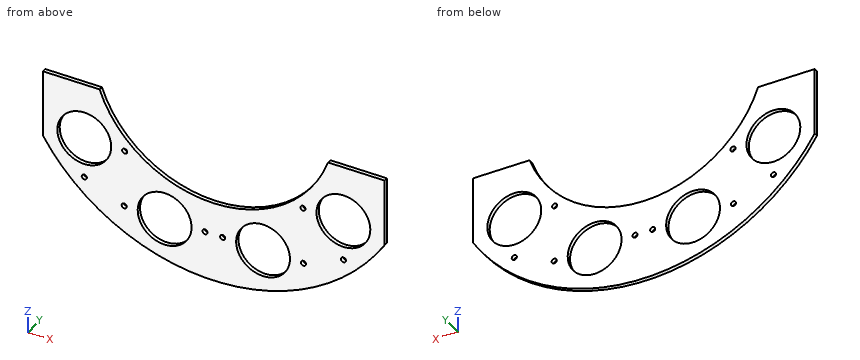
```python
from build123d import *

# Parameters (mm, degrees)
SKETCH3_R              = 20
BOSS_EXTRUDE3_DEPTH    = 3
F_10_24_TAPPED_HOLE1_D = 3.7973


with BuildPart() as part:
    # Sketch3 → Boss-Extrude3 (new body)
    with BuildSketch(Plane(origin=(0, 0, 0), x_dir=(1, 0, 0), z_dir=(0, 1, 0))):
        with BuildLine():
            Line((-126.885775404, -16.789832489), (-84.87168845, -16.789832489))
            ThreePointArc((-84.87168845, -16.789832489), (0, 43.227962976), (84.87168845, -16.789832489))
            Line((84.87168845, -16.789832489), (126.885775404, -16.789832489))
            Line((126.885775404, -16.789832489), (126.885775404, 33.210167511))
            ThreePointArc((126.885775404, 33.210167511), (0, 103.210167511), (-126.885775404, 33.210167511))
            Line((-126.885775404, 33.210167511), (-126.885775404, -16.789832489))
        make_face()
        with Locations(Location((-36.555626875, 67.506651026, 0), (0, 0, 270))):
            Circle(SKETCH3_R, mode=Mode.SUBTRACT)
        with Locations(Location((-96.223855306, 24.910723088, 0), (0, 0, 270))):
            Circle(SKETCH3_R, mode=Mode.SUBTRACT)
        with Locations(Location((36.555626875, 67.506651026, 0), (0, 0, 270))):
            Circle(SKETCH3_R, mode=Mode.SUBTRACT)
        with Locations(Location((96.223855306, 24.910723088, 0), (0, 0, 270))):
            Circle(SKETCH3_R, mode=Mode.SUBTRACT)
    extrude(amount=BOSS_EXTRUDE3_DEPTH)

    # #10-24 Tapped Hole1 (through all)
    with Locations(Plane(origin=(0, 3, 0), x_dir=(1, 0, 0), z_dir=(0, 1, 0))):
        with Locations((-66.223855306, 24.910723088), (-96.223855306, 54.910723088), (-66.555626875, 67.506651026), (-6.555626875, 67.506651026), (6.555626875, 67.506651026), (66.555626875, 67.506651026), (96.223855306, 54.910723088), (66.223855306, 24.910723088)):
            Hole(F_10_24_TAPPED_HOLE1_D / 2)


solid = part.part
```
CAD build for the part. Positions are in the model's coordinates, mm. Coordinates: 2 decimals unless noted, no trailing zeros. Loops run counter-clockwise (first coordinate to the right, second up) from the corner with the lowest first, then second, coordinate; pieces in that order, holes last. Notation, with made-up numbers: (-13.5, 47.25) - (-9.5, 47.25) arc R23 cw to (-9.5, 85.25) - close; hole circle Ø3 at (18, 84.25). An arc over 180 degrees is marked (long way). Use CSV: the item, a comma, the result in double quotes. Start each with the question number.
Q1. Cut at A-A, the plane x = -87.5. List the corners of the cut face in (y, z).
Q2. Cut at C-C, the plane z = -15. List the corners of the cut face in (x, y).
Q3. Drop flat-ended pins along their axis: P1, Ø1, axis at x = 52.5, y = 1.5, coming from the -Z side; P2, Ø3, axis at x = -96.22, z = -54.91, coming from the +Y side; P3, Ø1, axis at x = -91, y = 1.5, coming from the -Z side. Give the stop position or say it passes through.
Q4. Cut at D-D, the plane z = -72.5. List the corners of the cut face in (x, y).
Q5. Probe probe 1 along X at (y, z) = (2, -86); probe 2 along X at (y, z) = (0.75, -65); probe 3 along X at (y, z) = (1.9, -31.5). List the from-to ranges inside material, lowest first. Write a range as from..to.
Q6. Cut at B-B, the plane z = 1.5. List the corners of the cut face in (x, y).
Here are the results:
1,outline,"(0, -75.05) - (3, -75.05) - (3, -42.91) - (0, -42.91) - close; (0, -6.91) - (3, -6.91) - (3, 16.79) - (0, 16.79) - close"
2,outline,"(-126.89, 0) - (-113.6, 0) - (-113.6, 3) - (-126.89, 3) - close; (-78.85, 0) - (-65.46, 0) - (-65.46, 3) - (-78.85, 3) - close; (65.46, 0) - (78.85, 0) - (78.85, 3) - (65.46, 3) - close; (113.6, 0) - (126.89, 0) - (126.89, 3) - (113.6, 3) - close"
3,P1,"z = -93.91"
3,P2,"through"
3,P3,"z = -72.83"
4,outline,"(-90.94, 0) - (-55.92, 0) - (-55.92, 3) - (-90.94, 3) - close; (-17.19, 0) - (17.19, 0) - (17.19, 3) - (-17.19, 3) - close; (55.92, 0) - (90.94, 0) - (90.94, 3) - (55.92, 3) - close"
5,probe 1,"-69.76..-44.17, -28.94..28.94, 44.17..69.76"
5,probe 2,"-100.02..-56.4, -16.71..16.71, 56.4..100.02"
5,probe 3,"-126.89..-115.11, -77.34..-44.43, 44.43..77.34, 115.11..126.89"
6,outline,"(-126.89, 0) - (-77.79, 0) - (-77.79, 3) - (-126.89, 3) - close; (77.79, 0) - (126.89, 0) - (126.89, 3) - (77.79, 3) - close"
